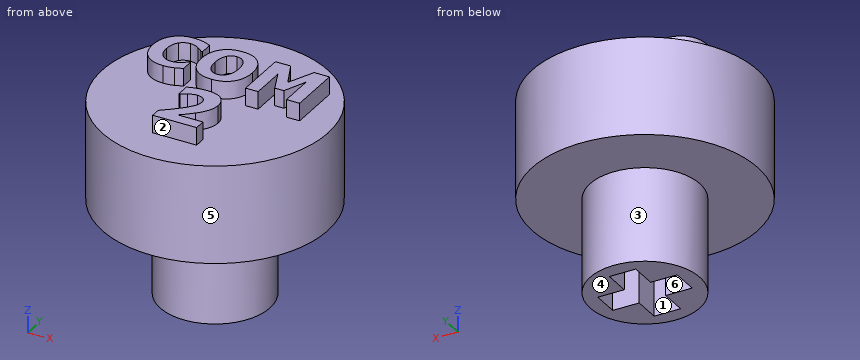
Autodesk Inventor part; units mm, degrees
ref_plane "YZ Plane" through (0, 0, 0) normal (1, 0, 0) x (0, 1, 0)
ref_plane "XZ Plane" through (0, 0, 0) normal (0, 1, 0) x (-1, 0, 0)
ref_plane "XY Plane" through (0, 0, 0) normal (0, 0, 1) x (1, 0, 0)
sketch "Sketch1" plane through (0, 0, 0) normal (0, 0, 1) x (1, 0, 0)
  circle A0 centre (0, 0) radius 6.22 construction
  circle A1 centre (0, 0) radius 2.8
  line L0 (-0.675, 0.675) -> (-0.675, 2.025)
  line L1 (-0.675, 2.025) -> (0.675, 2.025)
  line L2 (0.675, 2.025) -> (0.675, 0.675)
  line L3 (0.675, 0.675) -> (2.025, 0.675)
  line L4 (2.025, 0.675) -> (2.025, -0.675)
  line L5 (2.025, -0.675) -> (0.675, -0.675)
  line L6 (0.675, -0.675) -> (0.675, -2.025)
  line L7 (0.675, -2.025) -> (-0.675, -2.025)
  line L8 (-0.675, -2.025) -> (-0.675, -0.675)
  line L9 (-0.675, -0.675) -> (-2.025, -0.675)
  line L10 (-2.025, -0.675) -> (-2.025, 0.675)
  line L11 (-2.025, 0.675) -> (-0.675, 0.675)
  circle A2 centre (0, 0) radius 5.75
  point P0 (-6.07, -6.1)
  dimension "d0" = 12.44
  dimension "d1" = 0.47
extrude "Extrusion1" add sketch "Sketch1" along normal blind 5 contours A1 | L0 L1 L2 L3 L4 L5 L6 L7 L8 L9 L10 L11 | A2
extrude "Extrusion2" add sketch "Sketch1" against normal blind 4.8 contours A1
sketch "Sketch2" plane through (0, 0, 5) normal (0, 0, 1) x (1, 0, 0)
  point P0 (0, 0)
sketch "Sketch3" plane through (0, 0, 5) normal (0, 0, 1) x (1, 0, 0)
  line L0 (-4.2566, 3.1068) -> (4.2414, 3.1068) construction
  line L1 (4.2414, 3.1068) -> (4.2414, 0.2437) construction
  line L2 (4.2414, 0.2437) -> (-4.2566, 0.2437) construction
  line L3 (-4.2566, 0.2437) -> (-4.2566, 3.1068) construction
  line L4 (-1.3588, -0.6738) -> (1.3131, -0.6738) construction
  line L5 (1.3131, -0.6738) -> (1.3131, -3.7312) construction
  line L6 (1.3131, -3.7312) -> (-1.3588, -3.7312) construction
  line L7 (-1.3588, -3.7312) -> (-1.3588, -0.6738) construction
  spline S0 degree 2 poles (-2.8125, 0.2974) (-3.4208, 0.2974) (-4.1341, 1.0326) (-4.1341, 1.6977) knots 0 0 0 1 2 2 2
  spline S1 degree 2 poles (-4.1341, 1.6977) (-4.1341, 2.3388) (-3.4186, 3.1024) (-2.8103, 3.1024) knots 0 0 0 1 2 2 2
  spline S2 degree 2 poles (-2.8103, 3.1024) (-2.6506, 3.1024) (-2.3924, 3.0652) (-2.2743, 3.0346) knots 0 0 0 1 2 2 2
  spline S3 degree 2 poles (-2.2743, 3.0346) (-2.1824, 3.0062) (-1.9658, 2.9121) (-1.898, 2.8771) knots 0 0 0 1 2 2 2
  line L8 (-1.898, 2.8771) -> (-1.898, 2.2338)
  line L9 (-1.898, 2.2338) -> (-1.9658, 2.2338)
  spline S4 degree 2 poles (-1.9658, 2.2338) (-2.0161, 2.2775) (-2.1649, 2.4001) (-2.259, 2.457) knots 0 0 0 1 2 2 2
  spline S5 degree 2 poles (-2.259, 2.457) (-2.3531, 2.516) (-2.5784, 2.597) (-2.7031, 2.597) knots 0 0 0 1 2 2 2
  spline S6 degree 2 poles (-2.7031, 2.597) (-2.8497, 2.597) (-3.0926, 2.5051) (-3.2042, 2.3891) knots 0 0 0 1 2 2 2
  spline S7 degree 2 poles (-3.2042, 2.3891) (-3.3048, 2.2863) (-3.4339, 1.934) (-3.4339, 1.6955) knots 0 0 0 1 2 2 2
  spline S8 degree 2 poles (-3.4339, 1.6955) (-3.4339, 1.4439) (-3.3005, 1.1004) (-3.1911, 0.9954) knots 0 0 0 1 2 2 2
  spline S9 degree 2 poles (-3.1911, 0.9954) (-3.086, 0.8925) (-2.8279, 0.8028) (-2.6988, 0.8028) knots 0 0 0 1 2 2 2
  spline S10 degree 2 poles (-2.6988, 0.8028) (-2.5653, 0.8028) (-2.3224, 0.8925) (-2.2393, 0.9472) knots 0 0 0 1 2 2 2
  spline S11 degree 2 poles (-2.2393, 0.9472) (-2.1474, 1.0019) (-2.0095, 1.1179) (-1.9592, 1.1639) knots 0 0 0 1 2 2 2
  line L10 (-1.9592, 1.1639) -> (-1.898, 1.1639)
  line L11 (-1.898, 1.1639) -> (-1.898, 0.5293)
  spline S12 degree 2 poles (-1.898, 0.5293) (-1.9723, 0.4943) (-2.1671, 0.4068) (-2.2721, 0.3762) knots 0 0 0 1 2 2 2
  spline S13 degree 2 poles (-2.2721, 0.3762) (-2.399, 0.3368) (-2.62, 0.2974) (-2.8125, 0.2974) knots 0 0 0 1 2 2 2
  spline S14 degree 2 poles (0.9596, 1.6999) (0.9596, 1.0435) (0.2594, 0.293) (-0.3488, 0.293) knots 0 0 0 1 2 2 2
  spline S15 degree 2 poles (-0.3488, 0.293) (-0.9593, 0.293) (-1.6551, 1.0523) (-1.6551, 1.6999) knots 0 0 0 1 2 2 2
  spline S16 degree 2 poles (-1.6551, 1.6999) (-1.6551, 2.3498) (-0.9593, 3.1068) (-0.3488, 3.1068) knots 0 0 0 1 2 2 2
  spline S17 degree 2 poles (-0.3488, 3.1068) (0.2594, 3.1068) (0.9596, 2.3541) (0.9596, 1.6999) knots 0 0 0 1 2 2 2
  spline S18 degree 2 poles (0.2594, 1.6999) (0.2594, 1.9428) (0.161, 2.2819) (0.0756, 2.3891) knots 0 0 0 1 2 2 2
  spline S19 degree 2 poles (0.0756, 2.3891) (-0.0097, 2.5007) (-0.2285, 2.597) (-0.3467, 2.597) knots 0 0 0 1 2 2 2
  spline S20 degree 2 poles (-0.3467, 2.597) (-0.4714, 2.597) (-0.6749, 2.5073) (-0.7689, 2.3935) knots 0 0 0 1 2 2 2
  spline S21 degree 2 poles (-0.7689, 2.3935) (-0.8521, 2.2885) (-0.9549, 1.9406) (-0.9549, 1.6999) knots 0 0 0 1 2 2 2
  spline S22 degree 2 poles (-0.9549, 1.6999) (-0.9549, 1.4505) (-0.8565, 1.1223) (-0.7711, 1.0107) knots 0 0 0 1 2 2 2
  spline S23 degree 2 poles (-0.7711, 1.0107) (-0.6858, 0.8991) (-0.4648, 0.8028) (-0.3467, 0.8028) knots 0 0 0 1 2 2 2
  spline S24 degree 2 poles (-0.3467, 0.8028) (-0.2263, 0.8028) (-0.0031, 0.9057) (0.0778, 1.0151) knots 0 0 0 1 2 2 2
  spline S25 degree 2 poles (0.0778, 1.0151) (0.1653, 1.1332) (0.2594, 1.4461) (0.2594, 1.6999) knots 0 0 0 1 2 2 2
  line L12 (4.1191, 0.3499) -> (3.4452, 0.3499)
  line L13 (3.4452, 0.3499) -> (3.4452, 2.1397)
  line L14 (3.4452, 2.1397) -> (2.955, 0.9844)
  line L15 (2.955, 0.9844) -> (2.4912, 0.9844)
  line L16 (2.4912, 0.9844) -> (2.0011, 2.1397)
  line L17 (2.0011, 2.1397) -> (2.0011, 0.3499)
  line L18 (2.0011, 0.3499) -> (1.3622, 0.3499)
  line L19 (1.3622, 0.3499) -> (1.3622, 3.0499)
  line L20 (1.3622, 3.0499) -> (2.1433, 3.0499)
  line L21 (2.1433, 3.0499) -> (2.7428, 1.7174)
  line L22 (2.7428, 1.7174) -> (3.3379, 3.0499)
  line L23 (3.3379, 3.0499) -> (4.1191, 3.0499)
  line L24 (4.1191, 3.0499) -> (4.1191, 0.3499)
  line L25 (1.192, -3.7831) -> (-1.0498, -3.7831)
  line L26 (-1.0498, -3.7831) -> (-1.0498, -3.2863)
  spline S26 degree 2 poles (-1.0498, -3.2863) (-0.7656, -3.0589) (-0.3108, -2.6585) (-0.1402, -2.4781) knots 0 0 0 1 2 2 2
  spline S27 degree 2 poles (-0.1402, -2.4781) (0.0847, -2.2433) (0.2849, -1.8849) (0.2849, -1.697) knots 0 0 0 1 2 2 2
  spline S28 degree 2 poles (0.2849, -1.697) (0.2849, -1.4845) (0.0303, -1.2571) (-0.1971, -1.2571) knots 0 0 0 1 2 2 2
  spline S29 degree 2 poles (-0.1971, -1.2571) (-0.3133, -1.2571) (-0.5209, -1.3139) (-0.6272, -1.3584) knots 0 0 0 1 2 2 2
  spline S30 degree 2 poles (-0.6272, -1.3584) (-0.731, -1.4054) (-0.8793, -1.5043) (-0.9163, -1.529) knots 0 0 0 1 2 2 2
  line L27 (-0.9163, -1.529) -> (-0.9757, -1.529)
  line L28 (-0.9757, -1.529) -> (-0.9757, -0.8641)
  spline S31 degree 2 poles (-0.9757, -0.8641) (-0.8471, -0.8023) (-0.2984, -0.6738) (-0.0439, -0.6738) knots 0 0 0 1 2 2 2
  spline S32 degree 2 poles (-0.0439, -0.6738) (0.4999, -0.6738) (1.0585, -1.1582) (1.0585, -1.5957) knots 0 0 0 1 2 2 2
  spline S33 degree 2 poles (1.0585, -1.5957) (1.0585, -1.8651) (0.8039, -2.3842) (0.5098, -2.6808) knots 0 0 0 1 2 2 2
  spline S34 degree 2 poles (0.5098, -2.6808) (0.3244, -2.8637) (-0.0241, -3.1479) (-0.1007, -3.2072) knots 0 0 0 1 2 2 2
  line L29 (-0.1007, -3.2072) -> (1.192, -3.2072)
  line L30 (1.192, -3.2072) -> (1.192, -3.7831)
  point P0 (0, 0)
  point P1 (-0.0076, 0.2437)
  point P2 (-0.0228, -3.7312)
extrude "Extrusion3" add sketch "Sketch3" along normal blind 0.9
properties part number "IPC Com 2 key"
Can you work these out from the model? Positions are in its coordinate system, mm. Face numbers are marked on the shaded views. A direction names the side the tool comes from. Give positions to 0.01 mm unless a question says otherwise; leave off trailing zeros. Loops run counter-clockwise (first coordinate to the right, second up) from the corner with the lowest first, then second, coordinate; pieces in that order, holes last. Notation, with made-up numbers: M 26,-14.75 L 48,-14.75 A5 ccw 48,-10.75 Z; hole C -10,-19.5 d2. An arc over 180 degrees is marked long. Use one line per item in the form item = value. Start each with the question number.
(1) Thinking about a two-plate mould opening in Y: for the marked faces 1, 2, 3 and 4, which applies, released by +Y, released by -Y, zero draft, split by the parting line, or undercut?
(2) Please list where these lines run through material, in increasing order: line 1 (Z direction, x = 0, y = 3.5); line 2 (Y direction, x = 0.5, z = -3.75) (3 decimals); line 3 (Z direction, x = -0.25, y = 2.5).
(3) I want a section at A-A, the plane z = -2.5. Write out the boundary of the cut face in (x, y) (3 decimals), and give its area (3 significant figures).
(4) I'm going to push flat-ended pins straight in: P1, Ø1, axis at x = 2, z = -1, coming from the +Y side; P2, Ø0.7, axis at y = -1.5, z = -1.5, coming from the +X side; P3, Ø6, axis at x = -4.5, z = -1.5, coming from the +Y side. Where does each tip first touch, or does it pass through?
(5) I want a section at B-B, the plane z = 5.25. State how many separate pieces and enclosed holes the cut face has, and give its area (3 significant figures).
(6) I want a section at C-C, the plane y = 0. Write out the boundary of the cut face in (x, z) (3 decimals).
(7) On a 3-axis mill with a long thin cutter (end or side, diameter ignored), from which of +Z, -Z, +X, -X, +Y, -Y can I reach the whole of each face in a straight line? I mean the marked faces 5 and 6. Say none if no direction works.
(8) I want a section at D-D, the plane x = 4.5. Write out the boundary of the cut face in (y, z), and give its area (3 significant figures).
Worked out:
q1.face_1 = undercut
q1.face_2 = released by -Y
q1.face_3 = split by the parting line
q1.face_4 = zero draft
q2.line_1 = 0 to 5
q2.line_2 = -2.755 to -2.025, 2.025 to 2.755
q2.line_3 = -4.8 to 5
q3.outline = C 0,0 d5.6; hole M -2.025,-0.675 L -0.675,-0.675 L -0.675,-2.025 L 0.675,-2.025 L 0.675,-0.675 L 2.025,-0.675 L 2.025,0.675 L 0.675,0.675 L 0.675,2.025 L -0.675,2.025 L -0.675,0.675 L -2.025,0.675 Z
q3.area = 15.5 mm²
q4.P1 = 2.36
q4.P2 = 2.55
q4.P3 = 5.43
q5.separate_pieces = 4
q5.enclosed_holes = 1
q5.area = 16.5 mm²
q6.outline = M -5.75,0 L -2.8,0 L -2.8,-4.8 L -2.025,-4.8 L -2.025,0 L 2.025,0 L 2.025,-4.8 L 2.8,-4.8 L 2.8,0 L 5.75,0 L 5.75,5 L -5.75,5 Z
q7.face_5 = +Z, -Z
q7.face_6 = -Z
q8.outline = M -3.58,0 L 3.58,0 L 3.58,5 L -3.58,5 Z
q8.area = 35.8 mm²
